Print and shaded views of the part. All mm, measured from the part's lowest x, y and z. A direction names the side the tool comes from. Round coordinates to 2 decimals unless told otherwise and drop trailing zeros. Loops run counter-clockwise (first coordinate to the right, second up) from the corner with the lowest first, then second, coordinate; pieces in that order, holes last. Notation, with made-up numbers: (36.25, 54.25) - (82.25, 54.25) arc R19 cw to (82.25, 83.25) - close; hole circle Ø5 at (12, 62). An arc over 180 degrees is marked (long way). Put each result on its own line as item: value. Start each with the question number.
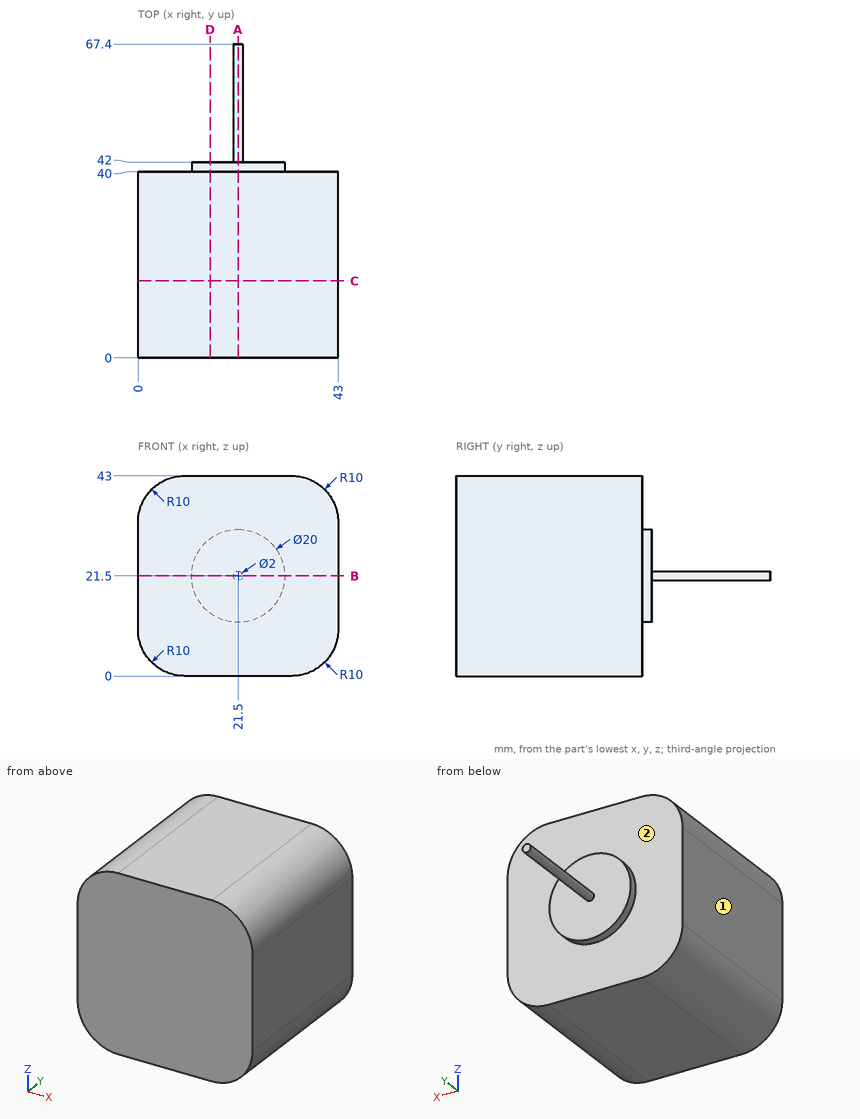
Item 1: Which spindle directions (+Z, -Z, +X, -X, +Y, -Y) get a long thin tool onto all of the face, cutting with end or side? Do the marked faces 1 and 2. Say none if no direction does.
Item 2: Slice it at A-A (x = 21.5). Give the cut face in (y, z), plus the area to 3 significant figures.
Item 3: Drill centre lines: probe 1 along Y at (x, z) = (16, 25); probe 2 along Y at (x, z) = (34, 13.5); probe 3 along Z at (x, y) = (36, 32). Where is each one in solid material? Low to high. Write a range as [from, to].
Item 4: Slice it at C-C (y = 16.5). Give the cut face in (x, z), plus the area to 3 significant figures.
Item 5: Slice it at B-B (z = 21.5). Give the cut face in (x, y).
Item 6: Slice it at D-D (x = 15.5). Give the cut face in (y, z), plus the area to 3 significant figures.
Item 7: Drop flat-ended pins along their axis: pin 1 Ø10 at (x, z) = (11, 24.5) entering from +Y; pin 2 Ø2 at (x, z) = (33, 5.5) entering from +Y; pin 3 Ø6 at (y, z) = (20.5, 38) entering from -X. Give the stop position or say it passes through.
Computed values:
1. face 1: +Z, -Z, -X, +Y, -Y
1. face 2: +Y
2. outline: (0, 0) - (40, 0) - (40, 11.5) - (42, 11.5) - (42, 20.5) - (67.4, 20.5) - (67.4, 22.5) - (42, 22.5) - (42, 31.5) - (40, 31.5) - (40, 43) - (0, 43) - close
2. area: 1,810 mm^2
3. probe 1: y = [0, 42]
3. probe 2: y = [0, 40]
3. probe 3: z = [0.46, 42.54]
4. outline: (0, 10) arc R10 ccw to (10, 0) - (33, 0) arc R10 ccw to (43, 10) - (43, 33) arc R10 ccw to (33, 43) - (10, 43) arc R10 ccw to (0, 33) - close
4. area: 1,760 mm^2
5. outline: (0, 0) - (43, 0) - (43, 40) - (31.5, 40) - (31.5, 42) - (22.5, 42) - (22.5, 67.4) - (20.5, 67.4) - (20.5, 42) - (11.5, 42) - (11.5, 40) - (0, 40) - close
6. outline: (0, 0) - (40, 0) - (40, 13.5) - (42, 13.5) - (42, 29.5) - (40, 29.5) - (40, 43) - (0, 43) - close
6. area: 1,750 mm^2
7. pin 1: stops at y = 42
7. pin 2: stops at y = 40
7. pin 3: stops at x = 0.2
